Input: part model. Units: mm. Frame: model coordinates. A direction names the side the tool comes from. Give positions to 0.01 mm unless a question says otherwise; leave off trailing zeros. Loops run counter-clockwise (first coordinate to the right, second up) from the corner with the lowest first, then second, coordinate; pieces in that order, holes last. Notation, with made-up numbers: M -14.5,-0.75 L 23.5,-0.75 A38 cw 23.5,38.25 Z; hole C 63,-4.5 d3. An arc over 180 degrees is marked long. One line per item, written item: value. Start each with the question number.
(1) Ray query, line 1 along Z through (x, y) = (30.5, 34); line 2 along Z through (x, y) = (28.5, 15); line 3 along Y through (x, z) = (38.5, 26.5). Return the intervals inside material, ascending. Write a range as from..to.
(2) Section B-B on y = 28.5. Output: boundary loops of the cut face in (x, z).
(3) Section D-D on y = 23.5. Output: boundary loops of the cut face in (x, z), plus the area to 3 significant figures.
(4) Section C-C on x = 16. Output: boundary loops of the cut face in (y, z).
(5) Access query for faces 1 (the flat face through (20, 30, 25)), 2 (the flat face through (20, 10, 35)), 3 (the flat face through (20, 30, 5)). Directions: +Z, -Z, +X, -X, +Y, -Y. A direction counts if a zero-diameter tool reaches every point of the face in a straight line with its end or side. Return the directions, or none.
(6) Section A-A on z = 8. Output: boundary loops of the cut face in (x, y), plus the area to 3 significant figures.
(7) Pin query (flat end, axial travel): P1, Ø5, axis at y = 12.5, z = 35, coming from the +X side; P2, Ø8, axis at y = 29, z = 23, coming from the -X side; P3, Ø1.5, axis at x = 28.5, y = 32.5, coming from the +Z side. Return the tip coordinate at first contact, or that it passes through.
```python
from build123d import *

# Parameters (mm, degrees)
SKETCH1_W           = 40
SKETCH1_H           = 40
BOSS_EXTRUDE1_DEPTH = 40
CUT_EXTRUDE1_DEPTH  = 40
SKETCH3_W           = 20
SKETCH3_H           = 10
CUT_EXTRUDE2_DEPTH  = 40
CUT_EXTRUDE3_DEPTH  = 20
CUT_EXTRUDE4_DEPTH  = 10


with BuildPart() as part:
    # Sketch1 → Boss-Extrude1 (new body)
    with BuildSketch(Plane.XY):
        with Locations((20, 20)):
            Rectangle(SKETCH1_W, SKETCH1_H)
    extrude(amount=BOSS_EXTRUDE1_DEPTH)

    # Sketch2 → Cut-Extrude1 (cut)
    with BuildSketch(Plane.XY.offset(40)):
        with BuildLine():
            Line((20, 40), (0, 40))
            Line((0, 40), (0, 20))
            ThreePointArc((0, 20), (5.857864376, 34.142135624), (20, 40))
        make_face()
        with BuildLine():
            ThreePointArc((20, 0), (5.857864376, 5.857864376), (0, 20))
            Line((0, 20), (0, 0))
            Line((0, 0), (20, 0))
        make_face()
        with BuildLine():
            Line((40, 0), (40, 20))
            ThreePointArc((40, 20), (34.142135624, 5.857864376), (20, 0))
            Line((20, 0), (40, 0))
        make_face()
        with BuildLine():
            Line((40, 40), (20, 40))
            ThreePointArc((20, 40), (34.142135624, 34.142135624), (40, 20))
            Line((40, 20), (40, 40))
        make_face()
    extrude(amount=-CUT_EXTRUDE1_DEPTH, mode=Mode.SUBTRACT)

    # Sketch3 → Cut-Extrude2 (cut)
    with BuildSketch(Plane(origin=(0, 0, 0), x_dir=(1, 0, 0), z_dir=(0, 1, 0))):
        with Locations((30, -35)):
            Rectangle(SKETCH3_W, SKETCH3_H)
    extrude(amount=CUT_EXTRUDE2_DEPTH, mode=Mode.SUBTRACT)

    # Sketch4 → Cut-Extrude3 (cut)
    with BuildSketch(Plane.XY.offset(40)):
        with BuildLine():
            Line((0, 20), (20, 20))
            Line((20, 20), (20, 40))
            ThreePointArc((20, 40), (5.857864376, 34.142135624), (0, 20))
        make_face()
    extrude(amount=-CUT_EXTRUDE3_DEPTH, mode=Mode.SUBTRACT)

    # Sketch5 → Cut-Extrude4 (cut)
    with BuildSketch(Plane(origin=(0, 0, 0), x_dir=(-1, 0, 0), z_dir=(0, 0, -1))):
        with BuildLine():
            Line((-40, 20), (-20, 20))
            Line((-20, 20), (-20, 40))
            ThreePointArc((-20, 40), (-34.142135624, 34.142135624), (-40, 20))
        make_face()
    extrude(amount=-CUT_EXTRUDE4_DEPTH, mode=Mode.SUBTRACT)


solid = part.part
```
Output values:
1. line 1: z = 10..30
1. line 2: z = 0..30
1. line 3: y = 12.4..27.6
2. outline: M 1.9,0 L 20,0 L 20,10 L 38.1,10 L 38.1,30 L 20,30 L 20,20 L 1.9,20 Z
3. outline: M 0.31,0 L 20,0 L 20,10 L 39.69,10 L 39.69,30 L 20,30 L 20,20 L 0.31,20 Z
3. area: 788 mm²
4. outline: M 0.4,0 L 39.6,0 L 39.6,20 L 20,20 L 20,40 L 0.4,40 Z
5. face 1: +Z, -X, +Y
5. face 2: +Z, +X, +Y, -Y
5. face 3: -Z, +X, +Y
6. outline: M 20,20 L 20,40 A20 ccw long 40,20 Z
6. area: 942 mm²
7. P1: stops at x = 20
7. P2: stops at x = 1.04
7. P3: stops at z = 30
